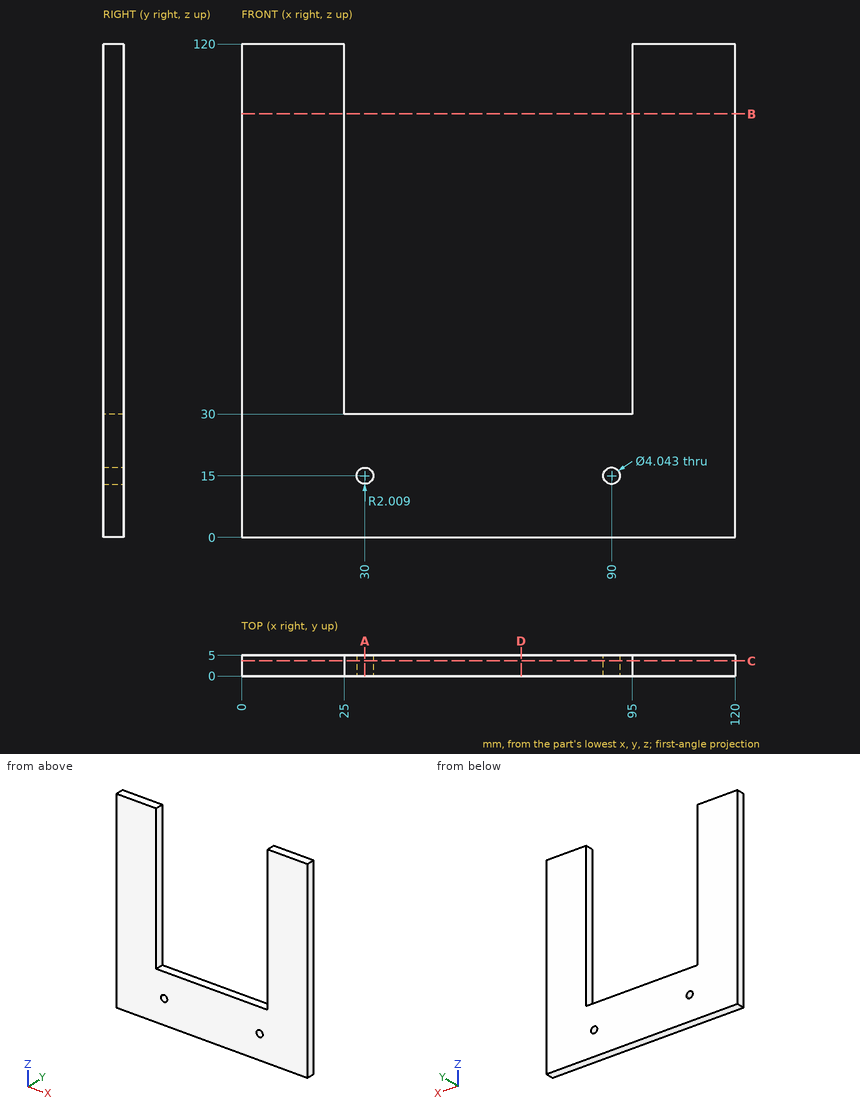
Part print with two shaded views. Sizes in mm from the minimum x, y, z corner. Give positions to 0.01 mm unless a question says otherwise; leave off trailing zeros. Order: outer loops, then holes, each group sorted by start corner. A loop starts at its lowest first (then second) coordinate and runs counter-clockwise, first axis right, second up. Notation, with made-up numbers: M 89.25,29.25 L 141.25,29.25 A19 cw 141.25,40.25 Z; hole C 80.25,72.5 d5. An arc over 180 degrees is marked long. Use one line per item in the form item = value.
1) Probe probe 1 along X at (y, z) = (2.4, 15); probe 2 along X at (y, z) = (1.6, 38); probe 3 along Z at (x, y) = (90, 1.25). List the from-to ranges inside material, lowest first.
Calculated:
probe_1 = 0 to 27.99, 32.01 to 87.98, 92.02 to 120
probe_2 = 0 to 25, 95 to 120
probe_3 = 0 to 12.98, 17.02 to 30
2) Saw through at D-D (x = 68). Give the cut face in (y, z).
Calculated:
outline = M 0,0 L 5,0 L 5,30 L 0,30 Z
3) Saw through at A-A (x = 30). Give the cut face in (y, z).
Calculated:
outline = M 0,0 L 5,0 L 5,12.99 L 0,12.99 Z; M 0,17.01 L 5,17.01 L 5,30 L 0,30 Z
4) Saw through at B-B (z = 103). Give the cut face in (x, y), plus the area to 3 significant figures.
Calculated:
outline = M 0,0 L 25,0 L 25,5 L 0,5 Z; M 95,0 L 120,0 L 120,5 L 95,5 Z
area = 250 mm2
5) Saw through at C-C (y = 3.7). Give the cut face in (x, z).
Calculated:
outline = M 0,0 L 120,0 L 120,120 L 95,120 L 95,30 L 25,30 L 25,120 L 0,120 Z; hole C 30,15 d4.02; hole C 90,15 d4.04
6) Drop a flat-ended pin along its axis: pin 1 (5.5 mm diameter, centred on x = 90, z = 15, fed in from -Y). Give the stop position or say it passes through.
Calculated:
pin_1 = 0
